```python
from build123d import *

# Parameters (mm, degrees)
SKETCH1_R               = 7.5
BOSS_EXTRUDE1_DEPTH     = 15
SKETCH2_R               = 7.5
BOSS_EXTRUDE2_DEPTH     = 50
SKETCH3_W               = 50
SKETCH3_H               = 40
BOSS_EXTRUDE3_DEPTH     = 65
CUT_EXTRUDE1_DEPTH      = 105.024035684
CUT_EXTRUDE2_DEPTH      = 96.372952141
BOSS_EXTRUDE7_START     = -15
SKETCH6_R               = 2
BOSS_EXTRUDE7_DEPTH     = 30
SKETCH8_W               = 15
SKETCH8_H               = 10
BOSS_EXTRUDE10_DEPTH    = 15
SKETCH9_R               = 4
CUT_EXTRUDE3_DEPTH      = 109.310895112
CUT_EXTRUDE6_DEPTH      = 20
ESQUISSE1_R             = 2
ENL_V_MAT_EXTRU_1_DEPTH = 10


with BuildPart() as part:
    # Sketch1 → Boss-Extrude1 (new body)
    with BuildSketch(Plane.XY):
        with BuildLine():
            Line((0, 0), (50, 0))
            Line((50, 0), (50, 50))
            ThreePointArc((50, 50), (40.582575695, 63.228756555), (25, 58.660254038))
            ThreePointArc((25, 58.660254038), (9.417424305, 63.228756555), (0, 50))
            Line((0, 50), (0, 0))
        make_face()
        with Locations((36, 50)):
            Circle(SKETCH1_R, mode=Mode.SUBTRACT)
        with Locations((14, 50)):
            Circle(SKETCH1_R, mode=Mode.SUBTRACT)
    extrude(amount=BOSS_EXTRUDE1_DEPTH)

    # Sketch2 → Boss-Extrude2 (add)
    with BuildSketch(Plane.XY.offset(15)):
        with BuildLine():
            Line((0, 50), (0, 0))
            Line((0, 0), (25, 0))
            Line((25, 0), (25, 50))
            ThreePointArc((25, 50), (12.5, 62.5), (0, 50))
        make_face()
        with Locations((14, 50)):
            Circle(SKETCH2_R, mode=Mode.SUBTRACT)
    extrude(amount=BOSS_EXTRUDE2_DEPTH)

    # Sketch3 → Boss-Extrude3 (add)
    with BuildSketch(Plane(origin=(0, 0, 0), x_dir=(-1, 0, 0), z_dir=(0, 0, -1))):
        with Locations((-25, 20)):
            Rectangle(SKETCH3_W, SKETCH3_H)
    extrude(amount=-BOSS_EXTRUDE3_DEPTH)

    # Sketch4 → Cut-Extrude1 (cut, through all)
    with BuildSketch(Plane.ZY):
        with BuildLine():
            Line((23, 36), (43, 36))
            ThreePointArc((43, 36), (53, 26), (43, 16))
            Line((43, 16), (23, 16))
            ThreePointArc((23, 16), (13, 26), (23, 36))
        make_face()
    extrude(amount=-CUT_EXTRUDE1_DEPTH, mode=Mode.SUBTRACT)

    # Sketch2_3 → Cut-Extrude2 (cut, through all)
    with BuildSketch(Plane.XY.offset(15)):
        with BuildLine():
            ThreePointArc((50, 50), (37.5, 62.5), (25, 50))
            ThreePointArc((25, 50), (12.5, 62.5), (0, 50))
            ThreePointArc((0, 50), (9.417424305, 63.228756555), (25, 58.660254038))
            ThreePointArc((25, 58.660254038), (40.582575695, 63.228756555), (50, 50))
        make_face()
    extrude(amount=-CUT_EXTRUDE2_DEPTH, mode=Mode.SUBTRACT)

    # Sketch6 → Boss-Extrude7 (add)
    with BuildSketch(Plane.XZ.offset(BOSS_EXTRUDE7_START)):
        Polygon((0, 65), (-15, 65), (-15, 47.450556951), (-8.979909906, 34.061546791), (-16.494563126, 21.450556951), (-36.494563126, 21.450556951), (-38.979909906, 25), (-60, 25), (-60, 16), (-56.169777784, 12.786061952), (-56.169777784, 0), (0, 0), align=None)
        with Locations(Location((-41.994563126, 16, 0), (0, 0, 270))):
            Circle(SKETCH6_R, mode=Mode.SUBTRACT)
        with Locations(Location((-10.994563126, 16, 0), (0, 0, 270))):
            Circle(SKETCH6_R, mode=Mode.SUBTRACT)
        with Locations(Location((-10.994563126, 47, 0), (0, 0, 270))):
            Circle(SKETCH6_R, mode=Mode.SUBTRACT)
    extrude(amount=-BOSS_EXTRUDE7_DEPTH)

    # Sketch8 → Boss-Extrude10 (add)
    with BuildSketch(Plane(origin=(0, 15, 0), x_dir=(-1, 0, 0), z_dir=(0, -1, 0))):
        with Locations((7.5, -60)):
            Rectangle(SKETCH8_W, SKETCH8_H)
        Polygon((60, -16), (60, -25), (50, -25), (50, -10), (0, -10), (0, 0), (56.169777784, 0), (56.169777784, -12.786061952), align=None)
    extrude(amount=BOSS_EXTRUDE10_DEPTH)

    # Sketch9 → Cut-Extrude3 (cut, through all)
    with BuildSketch(Plane.ZY):
        with Locations((58, 13)):
            Circle(SKETCH9_R)
        with Locations((7, 13)):
            Circle(SKETCH9_R)
    extrude(amount=-CUT_EXTRUDE3_DEPTH, mode=Mode.SUBTRACT)

    # Sketch10 → Cut-Extrude6 (cut)
    with BuildSketch(Plane(origin=(0, 0, 0), x_dir=(0, 0, -1), z_dir=(1, 0, 0))):
        with BuildLine():
            Line((-37, 33), (-27, 33))
            ThreePointArc((-27, 33), (-20, 26), (-27, 19))
            Line((-27, 19), (-37, 19))
            ThreePointArc((-37, 19), (-44, 26), (-37, 33))
        make_face()
    extrude(amount=-CUT_EXTRUDE6_DEPTH, mode=Mode.SUBTRACT)

    # Esquisse1 → Enl_v. mat.-Extru.1 (cut)
    with BuildSketch(Plane(origin=(0, 40, 0), x_dir=(1, 0, 0), z_dir=(0, 1, 0))):
        with Locations(Location((46, -42, 0), (0, 0, 270))):
            Circle(ESQUISSE1_R)
        with Locations(Location((46, -62, 0), (0, 0, 270))):
            Circle(ESQUISSE1_R)
    extrude(amount=-ENL_V_MAT_EXTRU_1_DEPTH, mode=Mode.SUBTRACT)


solid = part.part
```
Design review of the part built by this model. Coordinates are the model's own, in mm. A direction names the side the tool comes from. Give positions to 0.01 mm unless a question says otherwise; leave off trailing zeros. Write each loop counter-clockwise with the first axis right and the second up, starting at its lowest first coordinate (ties: lowest second). Pieces come first, ordered by that corner, then holes. Notation, with made-up numbers: (0.5, -25) - (24.5, -25) arc R33 ccw to (24.5, 6) - close; hole circle Ø6 at (38.25, -1). An arc over 180 degrees is marked (long way). Return JSON: item names as keys, results as strings. Group by question number.
(1) To check wall thickness, follow probe 1 along Y at (x, z) = (26.5, 41.5); probe 2 along Y at (x, z) = (40, 58); probe 3 along X at (y, z) = (14.5, 20). State the ranges of each line that lie inside material, in increasing order.
(2) We need section B-B, the plane x = -7. Give the boundary of the cut face in (y, z), then the cut area to 3 significant figures.
(3) We need section D-D, the plane x = 14. Give the boundary of the cut face in (y, z), then the cut area to 3 significant figures.
(4) We need section A-A, the plane y = 23. Give the boundary of the cut face in (x, z).
(5) Insertion check: pin 1 (2 mm diameter, centred on y = 11.5, z = 57, fed in from +X); pin 2 (13 mm diameter, centred on y = 13, z = 7, fed in from -X); pin 3 (1.5 mm diameter, centred on y = 43.5, z = 41.5, fed in from +X); pin 4 (3 mm diameter, centred on x = -25.5, y = 25.5, fed in from -Z). Each pin has a flat end and moves straight along its axis. Give the tip position at first contact, or say it passes through.
(6) Machinability: for faces 4 (the cylindrical face through (24.65, 16.966, 6.479)), 5 (the flat face through (-7, 8, 55)), 6 (the flat face through (-5, 19, 32)), 7 (the flat face through (-15, 28, 56)), 8 (the cylindrical face through (44, 35, 62)), which of the approach directions +Z, -Z, +X, -X, +Y, -Y give a long, thin tool a straight path to every point of the face, cutting with its end or side? Answer none if there is none.
(7) We need section C-C, the plane z = 7. Give the boundary of the cut face in (x, y).
(8) Mouldability with a two-part tool opening along Y and no side actions: class faces 1 (the flat face through (46, 30, 62)), 2 (the cylindrical face through (-8, 26, 20)), 3 (the flat face through (-49, 27, 25)) as +Y half, -Y half, draft (parallel to the pull), parting line (faces both ways), or undercut.
Reported:
{
 "1": {"probe 1": "y = 0 to 16, 36 to 40", "probe 2": "y = 0 to 9, 17 to 40", "probe 3": "x = -60 to -50, 0 to 50"},
 "2": {"outline": "(0, 0) - (45, 0) - (45, 65) - (0, 65) - (0, 55) - (15, 55) - (15, 10) - (0, 10) - close; hole (19, 27) arc R7 ccw to (33, 27) - (33, 37) arc R7 ccw to (19, 37) - close", "area": "1,960 mm2"},
 "3": {"outline": "(0, 0) - (42.5, 0) - (42.5, 65) - (0, 65) - close; (57.5, 0) - (62.41, 0) - (62.41, 65) - (57.5, 65) - close; hole circle Ø8 at (13, 7); hole circle Ø8 at (13, 58); hole (16, 23) arc R10 ccw to (36, 23) - (36, 43) arc R10 ccw to (16, 43) - close", "area": "2,270 mm2"},
 "4": {"outline": "(-60, 16) - (-56.17, 12.79) - (-56.17, 0) - (50, 0) - (50, 13.46) - (0, 13.46) - (0, 20.68) - (-20, 20.68) - (-20, 21.45) - (-36.49, 21.45) - (-38.98, 25) - (-60, 25) - close; (-15, 47.45) - (-13.14, 43.32) - (0, 43.32) - (0, 52.54) - (50, 52.54) - (50, 65) - (-15, 65) - close; hole circle Ø4 at (-41.99, 16); hole circle Ø4 at (-10.99, 16); hole circle Ø4 at (-10.99, 47)"},
 "5": {"pin 1": "stops at x = 0", "pin 2": "stops at x = -57.02", "pin 3": "stops at x = 25", "pin 4": "stops at z = 0"},
 "6": {"face 4": "+X", "face 5": "-X, -Y", "face 6": "+X, -X", "face 7": "+Z, -X, +Y, -Y", "face 8": "+Y"},
 "7": {"outline": "(-56.17, 0) - (50, 0) - (50, 9) - (0, 9) - (0, 17) - (50, 17) - (50, 50) arc R12.5 ccw to (25, 50) arc R12.5 ccw to (0, 50) - (0, 45) - (-56.17, 45) - close; hole circle Ø15 at (14, 50); hole circle Ø15 at (36, 50)"},
 "8": {"face 1": "+Y half", "face 2": "undercut", "face 3": "draft"}
}
